Work out the finished part from the listing and answer in its coordinate system (mm). A direction names the side the tool comes from. Round coordinates to 2 decimals unless told otherwise and drop trailing zeros. Loops run counter-clockwise (first coordinate to the right, second up) from the corner with the lowest first, then second, coordinate; pieces in that order, holes last. Notation, with made-up numbers: (7.25, 84) - (46.25, 84) arc R29 ccw to (46.25, 111) - close; hole circle Ø7 at (81, 44.25). An arc over 180 degrees is marked (long way). Answer as CSV lines item,"result". Start each with the question number.
```python
from build123d import *

# Parameters (mm, degrees)
F0_W     = 25.4
F0_H     = 12.7
F1_DEPTH = 1.27
F2_W     = 0.635
F2_H     = 0.635
F3_DEPTH = 12.7
F4_W     = 0.635
F4_H     = 0.635
F5_DEPTH = 12.7


with BuildPart() as f1:
    # F0 (on Top) → F1 (new body)
    with BuildSketch(Plane.XY):
        Rectangle(F0_W, F0_H)
    extrude(amount=F1_DEPTH)

    # F2 (on face) → F3 (join)
    with BuildSketch(Plane.XZ.offset(6.35)):
        with Locations((-11.7475, -0.3175)):
            Rectangle(F2_W, F2_H)
        with Locations((11.7475, -0.3175)):
            Rectangle(F2_W, F2_H)
    extrude(amount=-F3_DEPTH)

    # F4 (on face) → F5 (join)
    with BuildSketch(Plane(origin=(0, 0, -0.635), x_dir=(1, 0, 0), z_dir=(0, 0, -1))):
        with Locations((11.7475, -6.0325)):
            Rectangle(F4_W, F4_H)
        with Locations((11.7475, 6.0325)):
            Rectangle(F4_W, F4_H)
        with Locations((-11.7475, -6.0325)):
            Rectangle(F4_W, F4_H)
        with Locations((-11.7475, 6.0325)):
            Rectangle(F4_W, F4_H)
    extrude(amount=F5_DEPTH)


solid = f1.part
```
Item 1: Determine the mould class of faces 5 (the face through (-12.7, 0, 1)), 6 (the face through (0, 6.35, 1)), 7 (the face through (12.7, 0, 1)), 8 (the face through (-11.43, 0, -0.3)) for opening direction X: pulls with the +X half, pulls with the -X half, needs draft (parallel to the pull), parting line crosses it, or undercut.
Item 2: Flat-ended cylindrical pins translate along their axes: pin 1 Ø5 at (y, z) = (1, -11) entering from +X; pin 2 Ø1.5 at (x, y) = (0.5, 3.5) entering from -Z. Find the tip coordinate at first contact, or state that the pin passes through.
Item 3: Find the intervals of material crossed by L1, parallel to Y at x = -11.5, z = -4.5 (3 decimals); L2, parallel to X at y = 1, z = -0.5 (3 decimals); L3, parallel to Z at x = -5.5, y = 4.5, in increasing order.
Item 4: Section C-C, the plane x = -4.25 is taken. Give the vertices of the cut face in (y, z), and give its area (3 significant figures).
Item 5: Which of the six approach directions +Z, -Z, +X, -X, +Y, -Y give full straight-line access (tool end or side, diameter ignored) to faces 1 (the face through (0, 0, 1.27)), 2 (the face through (-12.065, 0, -0.3)), 3 (the face through (12.065, 0, -0.2)), 4 (the face through (11.43, 0, -0.2))?
Item 6: Section A-A, the plane z = -9 is taken. Give the vertices of the cut face in (x, y) (3 decimals).
Item 7: Section B-B, the plane y = 4.5 is taken. Give the vertices of the cut face in (x, z) (3 decimals), and give its area (3 significant figures).
Answer:
1,face 5,"pulls with the -X half"
1,face 6,"needs draft"
1,face 7,"pulls with the +X half"
1,face 8,"undercut"
2,pin 1,"passes through"
2,pin 2,"stops at z = 0"
3,L1,"y = -6.35 to -5.715, 5.715 to 6.35"
3,L2,"x = -12.065 to -11.43, 11.43 to 12.065"
3,L3,"z = 0 to 1.27"
4,outline,"(-6.35, 0) - (6.35, 0) - (6.35, 1.27) - (-6.35, 1.27) - close"
4,area,"16.1 mm²"
5,face 1,"+Z, +X, -X, +Y, -Y"
5,face 2,"-Z, -X, +Y, -Y"
5,face 3,"-Z, +X, +Y, -Y"
5,face 4,"-Z, +Y, -Y"
6,outline,"(-12.065, -6.35) - (-11.43, -6.35) - (-11.43, -5.715) - (-12.065, -5.715) - close; (-12.065, 5.715) - (-11.43, 5.715) - (-11.43, 6.35) - (-12.065, 6.35) - close; (11.43, -6.35) - (12.065, -6.35) - (12.065, -5.715) - (11.43, -5.715) - close; (11.43, 5.715) - (12.065, 5.715) - (12.065, 6.35) - (11.43, 6.35) - close"
7,outline,"(-12.7, 0) - (-12.065, 0) - (-12.065, -0.635) - (-11.43, -0.635) - (-11.43, 0) - (11.43, 0) - (11.43, -0.635) - (12.065, -0.635) - (12.065, 0) - (12.7, 0) - (12.7, 1.27) - (-12.7, 1.27) - close"
7,area,"33.1 mm²"
